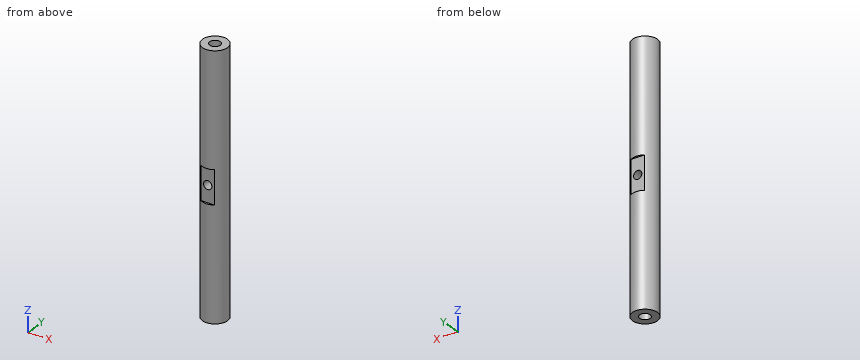
from build123d import *

# Parameters (mm, degrees)
SKETCH1_R           = 4.7625
BOSS_EXTRUDE1_DEPTH = 49.000000044
SKETCH4_W           = 12.7
SKETCH4_H           = 12.7
CUT_EXTRUDE1_DEPTH  = 0.762
SKETCH5_R           = 1.5875
CUT_EXTRUDE2_DEPTH  = 51.004715573


# Read off the part's stored shape, not the designer's step: #10-32 Tapped Hole1
with BuildPart() as part:
    # Sketch1 → Boss-Extrude1 (new, symmetric)
    with BuildSketch(Plane.XY):
        Circle(SKETCH1_R)
    extrude(amount=BOSS_EXTRUDE1_DEPTH, both=True)

    # #10-32 Tapped Hole1 outline → #10-32 Tapped Hole1 (revolve, cut)
    with BuildSketch(Plane.XZ):
        Polygon((2.0193, -36.970560044), (0, -35.757242196), (0, -49.000000044), (2.0193, -49.000000044), align=None)
        Polygon((0, 49.000000044), (0, 35.757242196), (2.0193, 36.970560044), (2.0193, 49.000000044), align=None)
    revolve(axis=Axis((0, 0, 0), (0, 0, 1)), mode=Mode.SUBTRACT)

    # Sketch4 → Cut-Extrude1 (cut)
    with BuildSketch(Plane(origin=(0, 4.7625, 0), x_dir=(1, 0, 0), z_dir=(0, 1, 0))):
        Rectangle(SKETCH4_W, SKETCH4_H)
    cut_extrude1 = extrude(amount=-CUT_EXTRUDE1_DEPTH, mode=Mode.SUBTRACT)

    # Sketch5 → Cut-Extrude2 (cut, through all)
    with BuildSketch(Plane(origin=(0, 4.0005, 0), x_dir=(1, 0, 0), z_dir=(0, 1, 0))):
        with Locations(Location((0, 0, 0), (0, 0, 270))):
            Circle(SKETCH5_R)
    extrude(amount=-CUT_EXTRUDE2_DEPTH, mode=Mode.SUBTRACT)

    # Mirror1: Cut-Extrude1 across plane
    add(cut_extrude1.mirror(Plane.ZX), mode=Mode.SUBTRACT)


solid = part.part
Check sheet for the modelled part. Datum: model origin and axes. Units: mm. Round coordinates to 2 decimals unless told otherwise and drop trailing zeros. Write each loop counter-clockwise with the first axis right and the second up, starting at its lowest first coordinate (ties: lowest second). Pieces come first, ordered by that corner, then holes. Notation, with made-up numbers: (11, 68) -> (57, 68) arc R13 cw to (57, 92) -> close; hole circle Ø8 at (-31, -13.75). An arc over 180 degrees is marked (long way). Answer as CSV lines item,"result". Start each with the question number.
1) Go/stop test with flat-tipped pins: P1, Ø3, axis at x = -3.5, z = 3.5, coming from the +Y side; P2, Ø1.5, axis at y = -2, z = 9, coming from the -X side; P3, Ø2.5, axis at x = -0.5, z = 1, coming from the -Y side; P4, Ø3, axis at x = 0, z = 0, coming from the -Y side. Record where each tip stops, or that it passes through.
2) Section check D-D on x = 3.5. Enter the section's corners in (y, z).
3) Section check C-C on z = 14.5. Enter the section's corners in (x, y) (1 decimal).
4) Material ranges on line 1 (Y direction, x = 0, z = -43.25); line 2 (Y direction, x = 4, z = -9.5); line 3 (X direction, y = 0.5, z = 0), recorded low to high. Write a range as from..to.
5) Section check B-B on z = -42. Enter the section's corners in (x, y) (1 decimal), and give its area (3 significant figures).
6) Section check A-A on z = 0. Enter the section's corners in (x, y) (1 decimal).
Found:
1,P1,"stops at y = 4"
1,P2,"stops at x = -4.6"
1,P3,"stops at y = -4"
1,P4,"passes through"
2,outline,"(-3.23, -49) -> (3.23, -49) -> (3.23, 49) -> (-3.23, 49) -> close"
3,outline,"circle Ø9.5 at (0, 0)"
4,line 1,"y = -4.76..-2.02, 2.02..4.76"
4,line 2,"y = -2.58..2.58"
4,line 3,"x = -4.74..-1.59, 1.59..4.74"
5,outline,"circle Ø9.5 at (0, 0); hole circle Ø4 at (0, 0)"
5,area,"58.4 mm^2"
6,outline,"(-2.6, -4) -> (-1.6, -4) -> (-1.6, 4) -> (-2.6, 4) arc R4.8 ccw to start; (1.6, -4) -> (2.6, -4) arc R4.8 ccw to (2.6, 4) -> (1.6, 4) -> close"
